Check sheet for the modelled part. Datum: model origin and axes. Units: mm. A direction names the side the tool comes from. Round coordinates to 2 decimals unless told otherwise and drop trailing zeros. Loops run counter-clockwise (first coordinate to the right, second up) from the corner with the lowest first, then second, coordinate; pieces in that order, holes last. Notation, with made-up numbers: (-16, -15.5) - (21, -15.5) arc R30 cw to (21, 9.5) - close; hole circle Ø7 at (76.5, 13). An arc over 180 degrees is marked (long way). Put each result on its own line as item: value. Start each with the question number.
Item 1: Section check B-B, the plane y = 12.5. Record the cut outline in (x, z), and give its area (3 significant figures).
Item 2: Draft check along Y on faces 4 (the flat face through (207.28, 138.09, 279.86)), 5 (the flat face through (108, 89, 270)), 6 (the flat face through (163.52, 143.815, 287.465)). Enter one of: pulls with the +Y half, pulls with the -Y half, needs draft (parallel to the pull), parting line crosses it, or undercut.
Item 3: Section check C-C, the plane z = 280. Give the number of separate pieces and of enclosed holes in the cut face, and give its area (3 significant figures).
Item 4: Material ranges on line 1 along Y through (x, z) = (168, 281); line 2 along Z through (x, y) = (194, 127); line 3 along X through (y, z) = (124.5, 284.25), recorded low to high.
Item 5: Section check A-A, the plane x = 15. Record the cut outline in (y, z), and give its area (3 significant figures).
Item 6: Section check D-D, the plane x = 55. Record the cut outline in (y, z), and give its area (3 significant figures).
Item 7: Tool access check on faces 1 (the cylindrical face through (152.577, 130.755, 273.451)), 2 (the flat face through (61.9, 24.92, 287.46)), 3 (the flat face through (0, 13, 280)). Record the directions out of +Z, -Z, +X, -X, +Y, -Y that give a thin tool (end or side, any length) a straight path to the whole face; none if there is none.
Item 8: Gauge pin test, flat ends, axial feed: pin 1 Ø5 at (x, y) = (168, 120.94) entering from -Z; pin 2 Ø2 at (y, z) = (40.5, 275.5) entering from +X; pin 3 Ø8 at (x, z) = (137, 272.5) entering from +Y. Record the tip position at first contact, or that the pin passes through.
Autodesk Inventor part; units mm, degrees
ref_plane "Work Plane1" through (164.5, 127, 270) normal (1, 0, 0) x (0, 0, 1)
ref_plane "XZ Plane" through (0, 0, 0) normal (0, 1, 0) x (-1, 0, 0)
ref_plane "XY Plane" through (0, 0, 0) normal (0, 0, 1) x (1, 0, 0)
sketch "Sketch1" plane through (0, 0, 0) normal (0, 0, 1) x (1, 0, 0)
  line L0 (0, 0) -> (100, 0)
  line L1 (100, 0) -> (100, 25)
  line L2 (100, 25) -> (0, 25)
  line L3 (0, 25) -> (0, 0)
  line L4 (0, 25) -> (115.2078, 140.2078)
  line L5 (100, 0) -> (177.7078, 77.7078)
  line L6 (151.2922, 176.2922) -> (200.5844, 163.0844)
  line L7 (200.5844, 163.0844) -> (213.7922, 113.7922)
  line L8 (213.7922, 113.7922) -> (177.7078, 77.7078)
  line L9 (177.7078, 77.7078) -> (128.4156, 90.9156)
  line L10 (128.4156, 90.9156) -> (115.2078, 140.2078)
  line L11 (115.2078, 140.2078) -> (151.2922, 176.2922)
  circle A0 centre (164.5, 127) radius 4
  dimension "d0" = 100
  dimension "d1" = 25
  dimension "d6" = 8
  dimension "d8" = 45
  dimension "d15" = 127
extrude "Extrusion1" add sketch "Sketch1" along normal blind 20
sketch "Sketch2" plane through (0, 0, 20) normal (0, 0, 1) x (1, 0, 0)
  line L0 (0, 25) -> (0, 0)
  line L1 (0, 0) -> (100, 0)
  line L2 (0, 25) -> (100, 25)
  line L3 (100, 25) -> (100, 0)
  line L4 (100, 0) -> (0, 0)
  line L5 (0, 0) -> (0, 25)
  line L6 (100, 25) -> (125, 25)
  line L7 (100, 0) -> (213.7922, 113.7922)
  line L8 (100, 0) -> (125, 25)
extrude "Extrusion2" add sketch "Sketch2" along normal blind 250
sketch "Sketch4" plane through (0, 0, 270) normal (0, 0, 1) x (1, 0, 0)
  line L0 (0, 25) -> (125, 25)
  line L1 (125, 25) -> (213.7922, 113.7922)
  line L2 (213.7922, 113.7922) -> (200.5844, 163.0844)
  line L3 (200.5844, 163.0844) -> (151.2922, 176.2922)
  line L4 (151.2922, 176.2922) -> (0, 25)
  circle A0 centre (164.5, 127) radius 4
  line L5 (100, 0) -> (125, 25)
  line L6 (125, 25) -> (0, 25)
  line L7 (0, 25) -> (0, 0)
  line L8 (0, 0) -> (100, 0)
extrude "Extrusion3" add sketch "Sketch4" along normal blind 20
sketch "Sketch5" plane through (0, 0, 0) normal (0, -1, 0) x (1, 0, 0)
  line L0 (0, 0) -> (100, 0)
  line L1 (100, 0) -> (100, 290)
  line L2 (0, 290) -> (100, 290)
  line L3 (0, 0) -> (0, 290)
  line L4 (0, 0) -> (-125.5737, 72.5)
  line L5 (-125.5737, 72.5) -> (-125.5737, 217.5)
  line L6 (-125.5737, 217.5) -> (0, 290)
  line L7 (0, 290) -> (125.5737, 217.5)
  line L8 (125.5737, 217.5) -> (125.5737, 72.5)
  line L9 (125.5737, 72.5) -> (0, 0)
  point P0 (0, 145)
extrude "Extrusion4" add sketch "Sketch5" against normal blind 25 contours L4 L5 L6 L3
sketch "Sketch6" plane through (0, 25, 20) normal (0, 1, 0) x (1, 0, 0)
  line L0 (100, 20) -> (100, -270)
  circle A0 centre (-24.528, -125) radius 3
  circle A1 centre (-31.528, -125) radius 1.5
  circle A2 centre (-21.028, -131.0622) radius 1.5
  circle A3 centre (-21.028, -118.9378) radius 1.5
  point P0 (0, 20)
  point P1 (100, -125)
  dimension "d18" = 6
  dimension "d19" = 124.528
  dimension "d20" = 3
  dimension "d21" = 7
  dimension "d24" = 360
extrude "Extrusion5" cut sketch "Sketch6" against normal through all
sketch "Sketch7" plane through (100, 0, 0) normal (0, -1, 0) x (1, 0, 0)
  circle A0 centre (-124.528, 145) radius 3
  circle A1 centre (-124.528, 145) radius 12
  point P0 (-100, 0)
  dimension "d28" = 24
extrude "Extrusion6" cut sketch "Sketch7" against normal blind 5
sketch "Sketch8" plane through (0, 0, 270) normal (0, 0, -1) x (-1, 0, 0)
  circle A0 centre (-164.5, 127) radius 4
  circle A1 centre (-164.5, 127) radius 12.5
  point P0 (0, 0)
  dimension "d31" = 25
extrude "Extrusion7" cut sketch "Sketch8" against normal blind 7
sketch "Sketch10" plane through (164.5, 127, 277) normal (0, 0, -1) x (-1, 0, 0)
  circle A0 centre (7, 0) radius 2
  circle A1 centre (0, 0) radius 4
  circle A2 centre (-3.5, 6.0622) radius 2
  circle A3 centre (-3.5, -6.0622) radius 2
  point P0 (164.5, -127)
  dimension "d34" = 4
  dimension "d37" = 360
  dimension "d39" = 7
extrude "Extrusion8" cut sketch "Sketch10" against normal through all
sketch "Sketch11" plane through (0, 0, 290) normal (0, 0, 1) x (1, 0, 0)
  circle A0 centre (168, 133.0622) radius 2
  circle A1 centre (164.5, 127) radius 4
  circle A2 centre (168, 133.0622) radius 4
  circle A3 centre (157.5, 127) radius 4
  circle A4 centre (168, 120.9378) radius 4
  point P0 (0, 0)
  dimension "d42" = 8
  dimension "d45" = 360
extrude "Extrusion9" cut sketch "Sketch11" against normal blind 3 contours A0 | A1 A4 A3 A2 | A2 A1 | A1 A2 | A4 A1 | A1 A4 | A3 A1 | A1 A3
ref_plane "Work Plane1" through (164.5, 127, 270) normal (1, 0, 0) x (0, 0, 1)
sketch "Sketch12" plane through (164.5, 127, 270) normal (1, 0, 0) x (0, 0, 1)
  line L0 (17, -1.9365) -> (17, 1.9365)
  line L1 (17, 1.9365) -> (20, 1.9365)
  line L2 (20, 3.9993) -> (20, 1.9365)
  line L3 (20, 3.9993) -> (17, 3.9993)
  line L4 (17, 3.9993) -> (17, 2.0628)
  line L5 (17, 2.0628) -> (20, 2.0628)
  line L6 (20, -2.0628) -> (20, 2.0628)
  line L7 (20, -2.0628) -> (17, -2.0628)
  line L8 (17, -2.0628) -> (17, -3.9993)
  line L9 (17, -3.9993) -> (20, -3.9993)
  line L10 (20, -1.9365) -> (20, -3.9993)
  line L11 (20, -1.9365) -> (17, -1.9365)
  line L12 (7, 4) -> (7, -4)
  line L13 (7, -12.5) -> (7, 12.5)
  line L14 (0, -12.5) -> (0, 12.5)
  circle A0 centre (3.5, 0) radius 2
  line L15 (0, -12.5) -> (7, -12.5)
  point P0 (-270, 127)
  point P1 (7, 0)
  point P2 (3.5, -12.5)
  dimension "d50" = 4
extrude "Extrusion10" cut sketch "Sketch12" along normal through all contours A0
sketch "Sketch13" plane through (0, 0, 270) normal (0, 0, -1) x (-1, 0, 0)
  circle A0 centre (-164.5, 127) radius 4
  line L0 (0, 0) -> (-100, 0)
  line L1 (0, 25) -> (0, 0)
  line L2 (-151.2922, 176.2922) -> (0, 25)
  line L3 (-200.5844, 163.0844) -> (-151.2922, 176.2922)
  line L4 (-213.7922, 113.7922) -> (-200.5844, 163.0844)
  line L5 (-100, 0) -> (-213.7922, 113.7922)
  line L6 (125.5737, 0) -> (0, 0)
  line L7 (125.5737, 0) -> (125.5737, 25)
  line L8 (0, 25) -> (125.5737, 25)
  line L9 (0, 25) -> (0, 0)
extrude "Extrusion11" cut sketch "Sketch13" along normal through all
sketch "Sketch14" plane through (0, 0, 270) normal (0, 0, -1) x (-1, 0, 0)
  line L0 (-151.2922, 176.2922) -> (0, 25)
  line L1 (0, 25) -> (0, 0)
  line L2 (0, 25) -> (0, 0)
  line L3 (0, 25) -> (34.641, 25)
  line L4 (34.641, 25) -> (34.641, 0)
  line L5 (34.641, 25) -> (0, 25)
  line L6 (0, 25) -> (34.641, 25)
  line L7 (34.641, 0) -> (-100, 0)
  line L8 (34.641, 25) -> (34.641, 0)
  line L9 (34.641, 0) -> (0, 0)
extrude "Extrusion12" cut sketch "Sketch14" against normal through all
sketch "Sketch15" plane through (0, 0, 290) normal (0, 0, 1) x (1, 0, 0)
  line L0 (15, 12.5) -> (90, 12.5) construction
  line L1 (0, 0) -> (100, 0)
  circle A0 centre (15, 12.5) radius 2.5
  circle A1 centre (90, 12.5) radius 2.5
  dimension "d57" = 12.5
  dimension "d58" = 10
  dimension "d59" = 75
  dimension "d60" = 5
  dimension "d61" = 5
extrude "Extrusion13" cut sketch "Sketch15" against normal through all
sketch "Sketch16" plane through (0, 0, 290) normal (0, 0, 1) x (1, 0, 0)
  arc A0 (167.9271, 124.9372) -> (167.9271, 129.0628) centre (164.5, 127) ccw
  circle A1 centre (164.5, 127) radius 26.5
  circle A2 centre (62.5, 40) radius 22.5
  line L0 (0, 25) -> (125, 25) construction
  line L1 (100, 0) -> (213.7922, 113.7922)
  line L2 (47.3944, 56.6755) -> (146.709, 146.64)
  line L3 (76.584, 22.4532) -> (181.0879, 106.3338)
  point P0 (0, 0)
  point P1 (62.5, 25)
  dimension "d64" = 53
  dimension "d65" = 45
  dimension "d67" = 15
extrude "Extrusion14" cut sketch "Sketch16" against normal blind 5
sketch "Sketch17" plane through (0, 0, 285) normal (0, 0, 1) x (1, 0, 0)
  line L0 (47.3944, 56.6755) -> (146.709, 146.64) construction
  line L1 (181.0879, 106.3338) -> (76.584, 22.4532) construction
  line L2 (97.0517, 101.6578) -> (128.8359, 64.3935) construction
  circle A0 centre (100.2965, 97.8536) radius 2.5
  circle A1 centre (125.5912, 68.1977) radius 2.5
  point P0 (0, 0)
  dimension "d70" = 5
  dimension "d71" = 5
  dimension "d72" = 5
  dimension "d73" = 5
extrude "Extrusion15" cut sketch "Sketch17" against normal through all
sketch "Sketch18" plane through (0, 0, 285) normal (0, 0, 1) x (1, 0, 0)
  arc A0 (181.0879, 106.3338) -> (146.709, 146.64) centre (164.5, 127) ccw
  line L0 (146.709, 146.64) -> (180.8089, 140.9105)
  line L1 (180.8089, 140.9105) -> (181.0879, 106.3338)
  arc A1 (47.3944, 56.6755) -> (76.584, 22.4532) centre (62.5, 40) ccw
  line L2 (62.5, 40) -> (180.8089, 140.9105)
  point P0 (0, 0)
  dimension "d76" = 100
extrude "Extrusion16" add sketch "Sketch18" along normal blind 5
sketch "Sketch19" plane through (0, 0, 290) normal (0, 0, 1) x (1, 0, 0)
  arc A0 (47.3944, 56.6755) -> (76.584, 22.4532) centre (62.5, 40) ccw
  line L0 (47.3944, 56.6755) -> (146.709, 146.64)
  line L1 (47.3944, 56.6755) -> (76.584, 22.4532)
  point P0 (0, 0)
  dimension "d0" = 100
extrude "Extrusion17" add sketch "Sketch19" against normal blind 5
sketch "Sketch20" plane through (0, 0, 285) normal (0, 0, 1) x (1, 0, 0)
  line L0 (47.3944, 56.6755) -> (76.584, 22.4532)
  circle A0 centre (164.5, 127) radius 4
  circle A1 centre (164.5, 127) radius 4
  line L1 (164.5, 127) -> (47.6313, 27.3179)
  line L2 (47.6313, 27.3179) -> (47.3944, 56.6755)
  line L3 (47.6313, 27.3179) -> (76.584, 22.4532)
  point P0 (0, 0)
  point P1 (61.9892, 39.5643)
  dimension "d81" = 100
extrude "Extrusion18" cut sketch "Sketch20" along normal through all contours L0 L1 L2 | L0 L3 L1
properties part number "HA02" material "ABS Plastic"
Check result:
1. outline: (0, 270) - (12.5, 270) - (12.5, 290) - (0, 290) - close; (17.5, 270) - (87.5, 270) - (87.5, 290) - (17.5, 290) - close; (92.5, 270) - (112.5, 270) - (112.5, 290) - (92.5, 290) - close
1. area: 2,050 mm²
2. face 4: pulls with the +Y half
2. face 5: needs draft
2. face 6: undercut
3. separate pieces: 1
3. enclosed holes: 8
3. area: 18,800 mm²
4. line 1: 68 to 118.94, 122.94 to 125.06, 128.94 to 131.06, 135.06 to 171.82
4. line 2: 270 to 271.5, 275.5 to 290
4. line 3: 99.5 to 161.38, 167.62 to 210.92
5. outline: (0, 270) - (10, 270) - (10, 290) - (0, 290) - close; (15, 270) - (40, 270) - (40, 290) - (15, 290) - close
5. area: 700 mm²
6. outline: (0, 270) - (80, 270) - (80, 290) - (63.57, 290) - (63.57, 285) - (26.08, 285) - (26.08, 290) - (0, 290) - close
6. area: 1,410 mm²
7. face 1: -Z
7. face 2: +Z
7. face 3: +Z, -Z, -X, +Y, -Y
8. pin 1: z = 277
8. pin 2: x = 141.5
8. pin 3: y = 166
